Can you work these out from the model? Positions are in its coordinate system, mm. Face numbers are marked on the shaded views. A direction names the side the tool comes from. Coordinates: 2 decimals unless noted, no trailing zeros. Write each loop counter-clockwise with the first axis right and the second up, starting at its lowest first coordinate (ties: lowest second). Pieces come first, ordered by that corner, then holes. Notation, with made-up numbers: (41.5, 55.25) - (57.5, 55.25) arc R37 ccw to (57.5, 91.25) - close; hole circle Ø10 at (-32, 76). An arc over 180 degrees is marked (long way). One line per question, with ' | ' between items. Start each with the question number.
from build123d import *

# Parameters (mm, degrees)
F0_W     = 20
F0_H     = 20
F1_DEPTH = 60
F2_W     = 40
F2_H     = 20
F3_DEPTH = 20
F4_W     = 20
F4_H     = 20
F5_DEPTH = 40
F6_W     = 20
F6_H     = 20
F7_DEPTH = 40
F8_W     = 20
F8_H     = 20
F9_DEPTH = 19.9


with BuildPart() as f1:
    # F0 (on Front) → F1 (new body)
    with BuildSketch(Plane.XZ):
        Rectangle(F0_W, F0_H)
    extrude(amount=F1_DEPTH)

    # F2 (on face) → F3 (join)
    with BuildSketch(Plane.YZ.offset(10)):
        with Locations((-20, 0)):
            Rectangle(F2_W, F2_H)
    extrude(amount=F3_DEPTH)

    # F4 (on face) → F5 (join)
    with BuildSketch(Plane(origin=(0, 0, -10), x_dir=(1, 0, 0), z_dir=(0, 0, -1))):
        with Locations((0, 50)):
            Rectangle(F4_W, F4_H)
    extrude(amount=F5_DEPTH)

    # F6 (on face) → F7 (join)
    with BuildSketch(Plane.YZ.offset(10)):
        with Locations((-50, -40)):
            Rectangle(F6_W, F6_H)
    extrude(amount=F7_DEPTH)

    # F8 (on face) → F9 (join)
    with BuildSketch(Plane.XY.offset(-30)):
        with Locations((40, -50)):
            Rectangle(F8_W, F8_H)
    extrude(amount=F9_DEPTH)


solid = f1.part
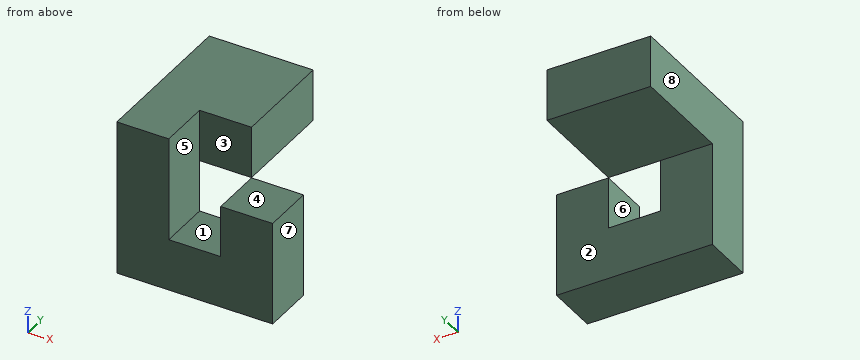
(1) Which directions (+Z, -Z, +X, -X, +Y, -Y) give clear straight access to the entire face, cutting with the end or side of a thin tool? Please do the marked faces 1, 2, 3, 4 and 5.
(2) If I drill on probe 1 along X at (y, z) = (-50.5, -19.5); probe 2 along Z at (x, y) = (12, -34); probe 3 along Y at (x, z) = (7, -44), over which ranges is the centre line in solid material (lowest first)?
(3) I'm going to push flat-ended pins straight in: pin 1 (20 mm diameter, centred on x = 6, y = -17, fed in from -Z); pin 2 (22 mm diameter, centred on x = 38, y = -50, fed in from +Z); pin 3 (8 mm diameter, centred on x = 29.5, y = -37, fed in from -Z); pin 4 (22 mm diameter, centred on y = -17.5, z = -2.5, fed in from +X). Where does each tip first touch, or does it pass through?
(4) If we section it at A-A on x = 28: List the corners of the cut face in (y, z) for me, plus the area to 3 significant figures.
(5) If we section it at B-B on z = -29: List the corners of the cut face in (x, y) for me.
(6) If we section it at C-C on y = -45.5: List the corners of the cut face in (x, z) for me.
(7) If we section it at D-D on x = 5.5: List the corners of the cut face in (y, z) for me.
(8) If we mould it in two halves opening along X, with no side actions, what happens to the marked faces 6, 7 and 8? For each: +X half, -X half, draft (parallel to the pull), parting line (faces both ways), or undercut.
Values:
1) face 1: +Z, +Y, -Y | face 2: -Z, +X, -X, +Y | face 3: +Z, +X, -Y | face 4: +Z, +X, +Y, -Y | face 5: +Z, -Y
2) probe 1: -10 to 10, 30 to 50 | probe 2: -10 to 10 | probe 3: -60 to -40
3) pin 1: z = -10 | pin 2: z = -10.1 | pin 3: z = -50 | pin 4: x = 30
4) outline: (-60, -50) - (-40, -50) - (-40, -30) - (-60, -30) - close; (-40, -10) - (0, -10) - (0, 10) - (-40, 10) - close | area: 1,200 mm2
5) outline: (-10, -60) - (10, -60) - (10, -40) - (-10, -40) - close; (30, -60) - (50, -60) - (50, -40) - (30, -40) - close
6) outline: (-10, -50) - (50, -50) - (50, -10.1) - (30, -10.1) - (30, -30) - (10, -30) - (10, 10) - (-10, 10) - close
7) outline: (-60, -50) - (-40, -50) - (-40, -10) - (0, -10) - (0, 10) - (-60, 10) - close
8) face 6: undercut | face 7: +X half | face 8: -X half
